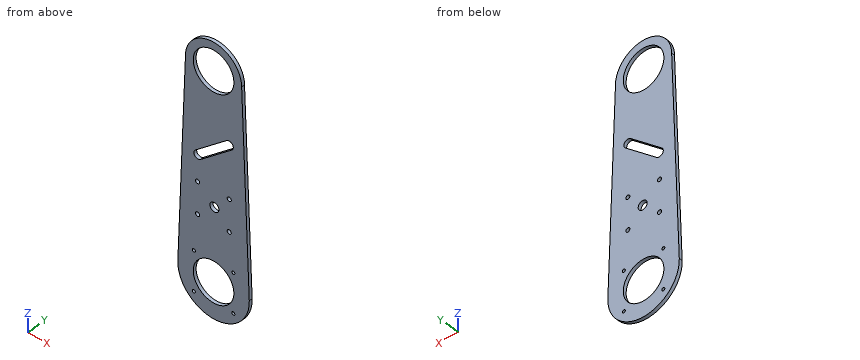
```python
from build123d import *

# Parameters (mm, degrees)
BOSS_EXTRUDE1_DEPTH     = 3.175
SKETCH2_R               = 19.9
CUT_EXTRUDE1_DEPTH      = 140.49939292
ESQUISSE2_R             = 1.5
ENL_V_MAT_EXTRU_1_DEPTH = 140.49939292
SKETCH3_R               = 4.425
CUT_EXTRUDE2_DEPTH      = 140.49939292
CUT_EXTRUDE4_DEPTH      = 140.49939292
SKETCH6_R               = 2
CUT_EXTRUDE5_DEPTH      = 140.49939292


with BuildPart() as part:
    # Sketch1 → Boss-Extrude1 (new body)
    with BuildSketch(Plane(origin=(0, 0, 0), x_dir=(1, 0, 0), z_dir=(0, 1, 0))):
        with BuildLine():
            Line((-27.5, -100), (-34.975254116, 98.684097441))
            ThreePointArc((-34.975254116, 98.684097441), (0, 135), (34.975254116, 98.684097441))
            Line((34.975254116, 98.684097441), (27.5, -100))
            ThreePointArc((27.5, -100), (0, -127.5), (-27.5, -100))
        make_face()
    extrude(amount=BOSS_EXTRUDE1_DEPTH)

    # Sketch2 → Cut-Extrude1 (cut, through all)
    with BuildSketch(Plane(origin=(0, 3.175, 0), x_dir=(1, 0, 0), z_dir=(0, 1, 0))):
        with Locations(Location((0, -100, 0), (0, 0, 270))):
            Circle(SKETCH2_R)
        with Locations(Location((0, 100, 0), (0, 0, 270))):
            Circle(SKETCH2_R)
    extrude(amount=-CUT_EXTRUDE1_DEPTH, mode=Mode.SUBTRACT)

    # Esquisse2 → Enlèv. mat.-Extru.1 (cut, through all)
    with BuildSketch(Plane(origin=(0, 3.175, 0), x_dir=(1, 0, 0), z_dir=(0, 1, 0))):
        with Locations(Location((19.339370465, 80.660629535, 0), (0, 0, 270))):
            Circle(ESQUISSE2_R)
        with Locations(Location((19.339370465, 119.339370465, 0), (0, 0, 270))):
            Circle(ESQUISSE2_R)
        with Locations(Location((-19.339370465, 119.339370465, 0), (0, 0, 270))):
            Circle(ESQUISSE2_R)
        with Locations(Location((-19.339370465, 80.660629535, 0), (0, 0, 270))):
            Circle(ESQUISSE2_R)
    extrude(amount=-ENL_V_MAT_EXTRU_1_DEPTH, mode=Mode.SUBTRACT)

    # Sketch3 → Cut-Extrude2 (cut, through all)
    with BuildSketch(Plane(origin=(0, 3.175, 0), x_dir=(1, 0, 0), z_dir=(0, 1, 0))):
        with Locations(Location((0.85, 28.7, 0), (0, 0, 270))):
            Circle(SKETCH3_R)
    extrude(amount=-CUT_EXTRUDE2_DEPTH, mode=Mode.SUBTRACT)

    # Sketch5 → Cut-Extrude4 (cut, through all)
    with BuildSketch(Plane(origin=(0, 3.175, 0), x_dir=(1, 0, 0), z_dir=(0, 1, 0))):
        with BuildLine():
            Line((12.749738424, -41.07568216), (-17.892039301, -15.364177772))
            ThreePointArc((-17.892039301, -15.364177772), (-18.385066635, -9.728849561), (-12.749738424, -9.235822228))
            Line((-12.749738424, -9.235822228), (17.892039301, -34.947326615))
            ThreePointArc((17.892039301, -34.947326615), (18.385066635, -40.582654826), (12.749738424, -41.07568216))
        make_face()
    extrude(amount=-CUT_EXTRUDE4_DEPTH, mode=Mode.SUBTRACT)

    # Sketch6 → Cut-Extrude5 (cut, through all)
    with BuildSketch(Plane(origin=(0, 0, 0), x_dir=(-1, 0, 0), z_dir=(0, -1, 0))):
        with Locations(Location((-15.35, 13.2, 0), (0, 0, 90))):
            Circle(SKETCH6_R)
        with Locations(Location((-15.35, 44.2, 0), (0, 0, 90))):
            Circle(SKETCH6_R)
        with Locations(Location((15.65, 44.2, 0), (0, 0, 90))):
            Circle(SKETCH6_R)
        with Locations(Location((15.65, 13.2, 0), (0, 0, 90))):
            Circle(SKETCH6_R)
    extrude(amount=-CUT_EXTRUDE5_DEPTH, mode=Mode.SUBTRACT)


solid = part.part
```
Design review of the part built by this model. Coordinates are the model's own, in mm. Coordinates: 2 decimals unless noted, no trailing zeros. Order: outer loops, then holes, each group sorted by start corner. A loop starts at its lowest first (then second) coordinate and runs counter-clockwise, first axis right, second up. Notation, with made-up numbers: (88, 52) - (141, 52) arc R25 ccw to (141, 75) - close; hole circle Ø10 at (20.25, -21.5). An arc over 180 degrees is marked (long way). Answer in a Markdown table with one row per item.
(1) Clearance check with flat-ended pins moving along their axes: pin 1 (3.5 mm diameter, centred on x = 19.34, z = -80.66, fed in from -Y); pin 2 (1.5 mm diameter, centred on x = 4.5, y = 1, fed in from +Z). State where each tip first meets the part, or that it passes through.
Checked values:
| item | result |
|---|---|
| pin 1 | y = 0 |
| pin 2 | z = 127.24 |
(2) Consider section B-B on y = 2.2. Give the number of separate pieces and of enclosed holes in the cut face, plus the area to 3 significant figures.
Checked values:
| item | result |
|---|---|
| separate pieces | 1 |
| enclosed holes | 12 |
| area | 12,600 mm^2 |
(3) Consider section A-A on z = 12.3. State the section outline as (x, y) points (3 decimals).
Checked values:
| item | result |
|---|---|
| outline | (-30.8, 0) - (-19.321, 0) - (-19.321, 3.175) - (-30.8, 3.175) - close; (-9.098, 0) - (30.8, 0) - (30.8, 3.175) - (-9.098, 3.175) - close |
(4) Wall thickness on line 1 along X through (y, z) = (0.35, -101); line 2 along Z through (x, y) = (12, 0.6); line 3 along X through (y, z) = (1.1, 100): over which ranges is each line inside the solid? List them lowest first. Write a range as from..to.
Checked values:
| item | result |
|---|---|
| line 1 | -34.99..-19.87, 19.87..34.99 |
| line 2 | -132.88..-115.87, -84.13..30, 40.45..84.13, 115.87..124.74 |
| line 3 | -27.5..-19.9, 19.9..27.5 |
(5) Consider section C-C on x = -31. State the section outline as (y, z) points (3 decimals), plus the area to 3 significant figures.
Checked values:
| item | result |
|---|---|
| outline | (0, -116.248) - (3.175, -116.248) - (3.175, 6.974) - (0, 6.974) - close |
| area | 391 mm^2 |
(6) Consider section D-D on z = -28.7. State the section outline as (x, y) points (3 decimals).
Checked values:
| item | result |
|---|---|
| outline | (-32.342, 0) - (-3.575, 0) - (-3.575, 3.175) - (-32.342, 3.175) - close; (5.275, 0) - (32.342, 0) - (32.342, 3.175) - (5.275, 3.175) - close |
